```python
from build123d import *

# Parameters (mm, degrees)
SKETCH_1_R          = 3.55
SKETCH_1_R_2        = 0.5
EXTRUDE_1_DEPTH     = 0.65
SKETCH_2_W          = 0.05
SKETCH_2_H          = 5.641200282
CUT_EXTRUDE_1_DEPTH = 8.092823177
FILLET_1_R          = 0.733333333
CUT_EXTRUDE_2_DEPTH = 8.092823177


with BuildPart() as part:
    # 草图1 → 凸台-拉伸1 (new body)
    with BuildSketch(Plane.XY):
        with BuildLine():
            Line((-1, -5.641200282), (1, -5.641200282))
            ThreePointArc((1, -5.641200282), (1.777817459, -5.319017741), (2.1, -4.541200282))
            Line((2.1, -4.541200282), (2.1, -3.394928957))
            ThreePointArc((2.1, -3.394928957), (0, 4.55), (-2.1, -3.394928957))
            Line((-2.1, -3.394928957), (-2.1, -4.541200282))
            ThreePointArc((-2.1, -4.541200282), (-1.777817459, -5.319017741), (-1, -5.641200282))
        make_face()
        Circle(SKETCH_1_R, mode=Mode.SUBTRACT)
        with Locations((-1, -4.541200282)):
            Circle(SKETCH_1_R_2, mode=Mode.SUBTRACT)
        with Locations(Location((1, -4.541200282, 0), (0, 0, 180))):
            Circle(SKETCH_1_R_2, mode=Mode.SUBTRACT)
    extrude(amount=EXTRUDE_1_DEPTH)

    # 草图2 → 切除-拉伸1 (cut, through all)
    with BuildSketch(Plane.XY.offset(0.65)):
        with Locations((0, -2.820600141)):
            Rectangle(SKETCH_2_W, SKETCH_2_H)
    extrude(amount=-CUT_EXTRUDE_1_DEPTH, mode=Mode.SUBTRACT)

    # 圆角1
    fillet_1_edges = [part.edges().sort_by_distance(p)[0] for p in [
        (-2.1, -3.394928957, 0.325),
        (2.1, -3.394928957, 0.325),
    ]]
    fillet(fillet_1_edges, radius=FILLET_1_R)

    # 草图3 → 切除-拉伸2 (cut, through all)
    with BuildSketch(Plane.XY.offset(0.65)):
        with BuildLine():
            Line((-1, -4.041200282), (1, -4.041200282))
            ThreePointArc((1, -4.041200282), (1.5, -4.541200282), (1, -5.041200282))
            Line((1, -5.041200282), (-1, -5.041200282))
            ThreePointArc((-1, -5.041200282), (-1.5, -4.541200282), (-1, -4.041200282))
        make_face()
    extrude(amount=-CUT_EXTRUDE_2_DEPTH, mode=Mode.SUBTRACT)


solid = part.part
```
Source: CAD feature listing. Evaluate the final solid. Frame: model axes, mm. Round coordinates to 2 decimals unless told otherwise and drop trailing zeros. Write each loop counter-clockwise with the first axis right and the second up, starting at its lowest first coordinate (ties: lowest second). Pieces come first, ordered by that corner, then holes. Notation, with made-up numbers: M 6,25.25 L 13,25.25 A22 cw 13,45.25 Z; hole C -17,69.25 d8. An arc over 180 degrees is marked long. Answer as a JSON object with one key per item and string values. Group by question number.
(1) Section query A-A on y = -4.25. Output: boundary loops of the cut face in (x, z).
(2) Section query B-B on x = -1.25. Output: boundary loops of the cut face in (y, z), then the cut area to 3 significant figures.
(3) Ray query, line 1 (X direction, y = -4.5, z = 0.55); line 2 (Y direction, x = 0.5, z = 0.35); line 3 (Y direction, x = 1.25, z = 0.6). Return the intervals inside material, ascending. Write a range as [from, to].
(4) Section query C-C on x = 3. Output: boundary loops of the cut face in (y, z).
Computed values:
{
 "1": {"outline": "M -2.1,0 L -1.41,0 L -1.41,0.65 L -2.1,0.65 Z; M 1.41,0 L 2.1,0 L 2.1,0.65 L 1.41,0.65 Z"},
 "2": {"outline": "M -5.61,0 L -4.97,0 L -4.97,0.65 L -5.61,0.65 Z; M -4.11,0 L -3.32,0 L -3.32,0.65 L -4.11,0.65 Z; M 3.32,0 L 4.36,0 L 4.36,0.65 L 3.32,0.65 Z", "area": "1.60 mm^2"},
 "3": {"line 1": "[-2.1, -1.5], [1.5, 2.1]", "line 2": "[-5.64, -5.04], [-4.04, -3.51], [3.51, 4.52]", "line 3": "[-5.61, -4.97], [-4.11, -3.32], [3.32, 4.36]"},
 "4": {"outline": "M -2.71,0 L -1.9,0 L -1.9,0.65 L -2.71,0.65 Z; M 1.9,0 L 3.31,0 L 3.31,0.65 L 1.9,0.65 Z"}
}
